Input: part model. Units: mm. Frame: model coordinates. A direction names the side the tool comes from. Coordinates: 2 decimals unless noted, no trailing zeros. Loops run counter-clockwise (first coordinate to the right, second up) from the corner with the lowest first, then second, coordinate; pieces in that order, holes last.
Item 1: Ray query, line 1 along X through (y, z) = (12.5, 1.3); line 2 along Y through (x, z) = (1, 0); line 3 along Y through (x, z) = (68.5, 1.1). Return the intervals inside material, ascending.
Item 2: Reachability of faces 1 (the flat face through (8.6, 9.14, 0.03)), 2 (the cylindrical face through (130.84, 13.4, 0.03)) from +Z, -Z, +X, -X, +Y, -Y: full face, straight path, thin tool, end or side. Return the list, or none.
Item 3: Section A-A on y = 0. Return loops of the section in (x, z), and give its area (3 significant figures).
Item 4: Section B-B on x = 15.5. Return loops of the section in (y, z), and give its area (3 significant figures).
Item 5: Pull-direction query (X, two-part tool) for faces 3 (the flat face through (73.3, 9.3, -2)), 4 (the flat face through (14.69, 2.57, 0.03)), 5 (the flat face through (8.871, 8.603, -0.028)); classes: released by +X, released by -X, zero draft, split by the parting line, or undercut.
Item 6: Contact query for flat-ended pins moving along their axis: P1, Ø1, axis at x = 20.5, y = 7, coming from the +Z side; P2, Ø1.5, axis at y = 13, z = 0, coming from the -X side. Output: stop coordinate, or through.
Item 7: Section C-C on z = 0.2. Return loops of the section in (x, y), and give its area (3 significant figures).
Autodesk Inventor part; units mm, degrees
ref_plane "Querschnittsebene" through (19.564749, 14.341157, 0) normal (-0.8925758, -0.4508975, 0) x (0, 0, 1)
ref_plane "Arbeitsebene2" through (21, 11.5, 0) normal (-1, 0, 0) x (0, 0, 1)
ref_plane "Arbeitsebene3" through (127.161065, 13.428, 0) normal (-0.9467755, 0.3218947, 0) x (0, 0, 1)
sketch "Skizzenpfad" plane through (0, 0, 0) normal (0, 0, 1) x (1, 0, 0)
  arc A0 (20.91835, 14.682051) -> (19.564749, 14.341157) centre (21, 11.5) ccw
  arc A1 (127.167049, 9.449131) -> (127.059003, 17.405564) centre (127.161065, 13.428) ccw
  arc A2 (27.996541, 9.299997) -> (26.970103, 9.056529) centre (28, 7) ccw
  arc A3 (-1.794064, 3.551446) -> (1.781665, -3.557682) centre (0, 0) ccw
  line L0 (-1.794064, 3.551446) -> (19.564749, 14.341157)
  line L1 (20.91835, 14.682051) -> (127.059003, 17.405564)
  line L2 (127.167049, 9.449131) -> (27.996541, 9.299997)
  line L3 (26.970103, 9.056529) -> (1.781665, -3.557682)
ref_plane "Querschnittsebene" through (19.564749, 14.341157, 0) normal (-0.8925758, -0.4508975, 0) x (0, 0, 1)
ref_plane "Arbeitsebene2" through (21, 11.5, 0) normal (-1, 0, 0) x (0, 0, 1)
ref_plane "Arbeitsebene3" through (127.161065, 13.428, 0) normal (-0.9467755, 0.3218947, 0) x (0, 0, 1)
ref_plane "Arbeitsebene4" through (0, 0, 0) normal (0.9748553, 0.2228388, 0) x (0, 0, 1)
sketch "Querschnitt" plane through (19.564749, 14.341157, 0) normal (-0.8925758, -0.4508975, 0) x (0, 0, 1)
  line L0 (-2, 0.3) -> (2, 0.3)
  line L1 (2, 0.3) -> (2, -0.3)
  line L2 (2, -0.3) -> (-2, -0.3)
  line L3 (-2, -0.3) -> (-2, 0.3)
  line L4 (-2, 0) -> (2, 0) construction
  point P0 (0, 0)
  point P1 (0, 0)
  dimension "d0" = 4
  dimension "d4" = 0.3
  dimension "d5" = 0.3
sweep "Riemen" add profiles "Querschnitt" path "Skizzenpfad"
equation "\"d0\" = da_B"
equation "\"d4\" = da_a"
equation "\"d5\" = da_a2"
equation "\"da_B\" = 4"
equation "\"da_pb\" = 2.5"
equation "\"da_L\" = 285"
equation "\"da_a\" = 0.3"
equation "\"da_S\" = 1.5"
equation "\"da_Beta\" = 20deg"
equation "\"da_Ht\" = 0.7"
equation "\"da_H\" = 1.3"
equation "\"da_a2\" = 0.3"
properties part number "Zahnriemen" material "Rubber"
Results found:
1. line 1: x = 15.25 to 16.59, 130.72 to 131.34
1. line 2: y = -4.16 to -3.54, 4.63 to 5.3
1. line 3: y = 9.06 to 9.66, 15.6 to 16.2
2. face 1: +Z, -Z, -X, +Y
2. face 2: +Z, -Z
3. outline: (-4.28, -2) - (-3.68, -2) - (-3.68, 2) - (-4.28, 2) - close; (8.22, -2) - (9.56, -2) - (9.56, 2) - (8.22, 2) - close
3. area: 7.76 mm2
4. outline: (2.98, -2) - (3.65, -2) - (3.65, 2) - (2.98, 2) - close; (11.95, -2) - (12.62, -2) - (12.62, 2) - (11.95, 2) - close
4. area: 5.37 mm2
5. face 3: zero draft
5. face 4: released by +X
5. face 5: undercut
6. P1: passes through
6. P2: stops at x = 14.76
7. outline: (-1.93, 3.82) arc R4.28 ccw to (1.92, -3.83) - (27.1, 8.79) arc R2 cw to (28, 9) - (127.17, 9.15) arc R4.28 ccw (long way) to (127.05, 17.71) - (20.91, 14.98) arc R3.48 ccw to (19.43, 14.61) - close; hole (-1.66, 3.28) arc R3.68 ccw to (1.65, -3.29) - (26.84, 9.32) arc R2.6 cw to (28, 9.6) - (127.17, 9.75) arc R3.68 ccw (long way) to (127.07, 17.11) - (20.93, 14.38) arc R2.88 ccw to (19.7, 14.07) - close
7. area: 171 mm2
